Here's how the part is built. I have some questions about the finished solid (model axes, mm). Face numbers are marked on the shaded views. A direction names the side the tool comes from. Give positions to 0.01 mm unless a question says otherwise; leave off trailing zeros. Order: outer loops, then holes, each group sorted by start corner. A loop starts at its lowest first (then second) coordinate and runs counter-clockwise, first axis right, second up. Notation, with made-up numbers: (11.5, 43.25) - (53.5, 43.25) arc R10 cw to (53.5, 52.25) - close; hole circle Ø7 at (42.5, -40). An arc over 180 degrees is marked (long way). One line per question, with ' | ' between items.
from build123d import *

# Parameters (mm, degrees)
ESQUISSE1_R                  = 19
BASE_EXTRUSION_DEPTH         = 18
ESQUISSE2_R                  = 13
ENL_V_MAT_EXTRU_1_DEPTH      = 14
ESQUISSE3_R                  = 8
ENL_V_MAT_EXTRU_2_DEPTH      = 19
ESQUISSE4_R                  = 1.25
ENL_V_MAT_EXTRU_3_DEPTH      = 19
R_P_TITION_CIRCULAIRE1_COUNT = 3
ESQUISSE5_R                  = 13
ENL_V_MAT_EXTRU_4_DEPTH      = 2
ESQUISSE6_R                  = 18.25
ENL_V_MAT_EXTRU_5_DEPTH      = 1
ESQUISSE7_R                  = 17
ENL_V_MAT_EXTRU_6_DEPTH      = 10
ESQUISSE8_R                  = 17.185
ENL_V_MAT_EXTRU_7_DEPTH      = 4
ESQUISSE9_R                  = 18.25
ENL_V_MAT_EXTRU_8_DEPTH      = 1
CHANFREIN1_SIZE              = 2
CHANFREIN2_SIZE              = 0.5


with BuildPart() as part:
    # Esquisse1 → Base-Extrusion (new body)
    with BuildSketch(Plane.XY):
        Circle(ESQUISSE1_R)
    extrude(amount=BASE_EXTRUSION_DEPTH)

    # Esquisse2 → Enlèv. mat.-Extru.1 (cut)
    with BuildSketch(Plane.XY.offset(18)):
        Circle(ESQUISSE2_R)
    extrude(amount=-ENL_V_MAT_EXTRU_1_DEPTH, mode=Mode.SUBTRACT)

    # Esquisse3 → Enlèv. mat.-Extru.2 (cut, through all)
    with BuildSketch(Plane(origin=(0, 0, 0), x_dir=(-1, 0, 0), z_dir=(0, 0, -1))):
        Circle(ESQUISSE3_R)
    extrude(amount=-ENL_V_MAT_EXTRU_2_DEPTH, mode=Mode.SUBTRACT)

    # Esquisse4 → Enlèv. mat.-Extru.3 (cut, through all)
    with BuildSketch(Plane(origin=(0, 0, 0), x_dir=(-1, 0, 0), z_dir=(0, 0, -1))):
        with Locations((0, 10.75)):
            Circle(ESQUISSE4_R)
    enl_v_mat_extru_3 = extrude(amount=-ENL_V_MAT_EXTRU_3_DEPTH, mode=Mode.SUBTRACT)

    # Répétition circulaire1: Enlèv. mat.-Extru.3 ×3 about axis
    r_p_tition_circulaire1_axis = Axis((0, 0, 0), (0, 0, -1))
    for i in range(1, R_P_TITION_CIRCULAIRE1_COUNT):
        add(enl_v_mat_extru_3.rotate(r_p_tition_circulaire1_axis, i * 360 / R_P_TITION_CIRCULAIRE1_COUNT), mode=Mode.SUBTRACT)

    # Esquisse5 → Enlèv. mat.-Extru.4 (cut)
    with BuildSketch(Plane.XY.offset(4)):
        Circle(ESQUISSE5_R)
    extrude(amount=-ENL_V_MAT_EXTRU_4_DEPTH, mode=Mode.SUBTRACT)

    # Esquisse6 → Enlèv. mat.-Extru.5 (cut)
    with BuildSketch(Plane.XY.offset(18)):
        Circle(ESQUISSE6_R)
    extrude(amount=-ENL_V_MAT_EXTRU_5_DEPTH, mode=Mode.SUBTRACT)

    # Esquisse7 → Enlèv. mat.-Extru.6 (cut, through all)
    with BuildSketch(Plane.XY.offset(9)):
        Circle(ESQUISSE7_R)
    extrude(amount=ENL_V_MAT_EXTRU_6_DEPTH, mode=Mode.SUBTRACT)

    # Esquisse8 → Enlèv. mat.-Extru.7 (cut)
    with BuildSketch(Plane.XY.offset(18)):
        Circle(ESQUISSE8_R)
    extrude(amount=-ENL_V_MAT_EXTRU_7_DEPTH, mode=Mode.SUBTRACT)

    # Esquisse9 → Enlèv. mat.-Extru.8 (cut)
    with BuildSketch(Plane.XY.offset(14)):
        Circle(ESQUISSE9_R)
    extrude(amount=ENL_V_MAT_EXTRU_8_DEPTH, mode=Mode.SUBTRACT)

    # Chanfrein1
    chanfrein1_edges = [part.edges().sort_by_distance(p)[0] for p in [
        (-19, 0, 0),
    ]]
    chamfer(chanfrein1_edges, length=CHANFREIN1_SIZE)

    # Chanfrein2
    chanfrein2_edges = [part.edges().sort_by_distance(p)[0] for p in [
        (-19, 0, 18),
    ]]
    chamfer(chanfrein2_edges, length=CHANFREIN2_SIZE)


solid = part.part
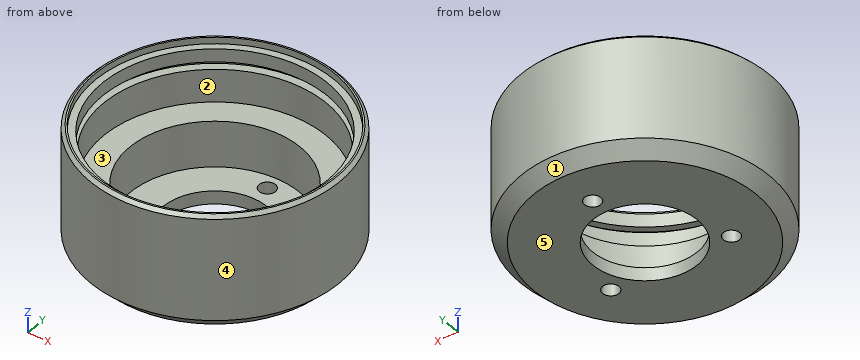
1) I'm going to push flat-ended pins straight in: P1, Ø9.5, axis at x = 0, y = 0, coming from the -Z side; P2, Ø3, axis at x = -11, z = 13, coming from the +Y side; P3, Ø11, axis at x = -6.5, y = -1, coming from the +Z side; P4, Ø5, axis at x = -3, z = 11, coming from the -Y side. Where does each tip first touch, or does it pass through?
Model answer:
P1: passes through | P2: stops at y = 16.45 | P3: stops at z = 2 | P4: stops at y = -18.99
2) Please list where these lines run through material, in increasing order: L1, parallel to Y at x = 0, z = 0.85; L2, parallel to Y at x = 0, z = 1; L3, parallel to Y at x = 0, z = 10.1.
Model answer:
L1: y = -17.85 to -8, 8 to 9.5, 12 to 17.85 | L2: y = -18 to -8, 8 to 9.5, 12 to 18 | L3: y = -19 to -17, 17 to 19
3) Thinking about a two-plate mould opening in X: for the marked faces 3, 4 and 5, which applies, +X half, -X half, draft (parallel to the pull), parting line (faces both ways), or undercut?
Model answer:
face 3: undercut | face 4: parting line | face 5: draft
4) I want a section at D-D (z = 1.5). List the corners of the cut face in (x, y) for me (3 decimals), plus the area to 3 significant figures.
Model answer:
outline: circle Ø37 at (0, 0); hole circle Ø2.5 at (-9.31, -5.375); hole circle Ø16 at (0, 0); hole circle Ø2.5 at (0, 10.75); hole circle Ø2.5 at (9.31, -5.375) | area: 859 mm2
5) On a 3-axis mill with a long thin cutter (end or side, diameter ignored), from which of +Z, -Z, +X, -X, +Y, -Y can I reach the whole of each face in a straight line? I mean the marked faces 1 and 2. Say none if no direction works.
Model answer:
face 1: -Z | face 2: +Z
6) I want a section at C-C (x = 0). State how many separate pieces and enclosed holes the cut face has, plus the area to 3 significant figures.
Model answer:
separate pieces: 3 | enclosed holes: 0 | area: 149 mm2
7) I want a section at B-B (z = 10). List the corners of the cut face in (x, y) for me, plus the area to 3 significant figures.
Model answer:
outline: circle Ø38 at (0, 0); hole circle Ø34 at (0, 0) | area: 226 mm2
